Verification items for the finished model (mm, model axes). Face numbers are marked on the shaded views. Round coordinates to 2 decimals unless told otherwise and drop trailing zeros. Loops run counter-clockwise (first coordinate to the right, second up) from the corner with the lowest first, then second, coordinate; pieces in that order, holes last. Notation, with made-up numbers: M -32,24 L 6,24 A19 ccw 6,35 Z; hole C 39,-28 d6. An arc over 180 degrees is marked long. One line per item, written item: value.
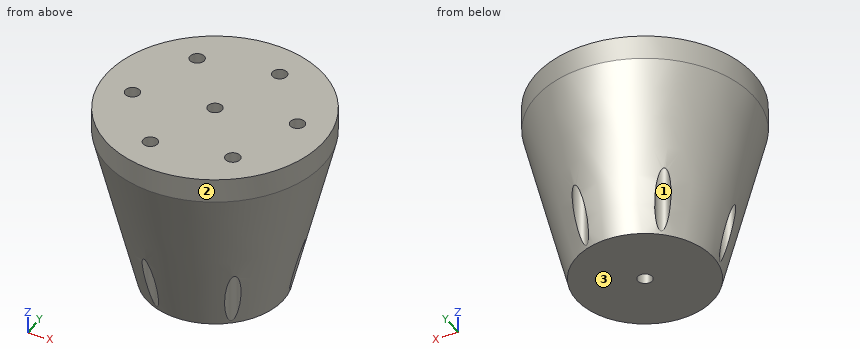
from build123d import *

# Parameters (mm, degrees)
F0_R     = 13.5
F0_R_2   = 0.9
F1_DEPTH = 23


# Not quite as in the source:
# - a fillet or chamfer that OpenCascade refuses, or shapes differently, is made with other operations: its cross-section is extruded or revolved along the edge and cut away or added


with BuildPart() as f1:
    # F0 (on Top) → F1 (new body)
    with BuildSketch(Plane.XY):
        Circle(F0_R)
        with Locations((-3.1211513103, -8.9726481319)):
            Circle(F0_R_2, mode=Mode.SUBTRACT)
        with Locations((-9.3311168766, -1.7833277421)):
            Circle(F0_R_2, mode=Mode.SUBTRACT)
        with Locations((6.2099655662, -7.1893203897)):
            Circle(F0_R_2, mode=Mode.SUBTRACT)
        with Locations((-6.2099655662, 7.1893203897)):
            Circle(F0_R_2, mode=Mode.SUBTRACT)
        Circle(F0_R_2, mode=Mode.SUBTRACT)
        with Locations((9.3311168766, 1.7833277421)):
            Circle(F0_R_2, mode=Mode.SUBTRACT)
        with Locations((3.1211513103, 8.9726481319)):
            Circle(F0_R_2, mode=Mode.SUBTRACT)
    extrude(amount=F1_DEPTH)

    # F2: chamfer of 20 x 5 on 1 edges, made by hand

    # F2_s1 → F2_t2 (revolve, cut)
    with BuildSketch(Plane.XZ):
        Polygon((13.5, 20), (8.5, 0), (13.5, 0), align=None)
    revolve(axis=Axis((0, 0, 0), (0, 0, 1)), mode=Mode.SUBTRACT)


solid = f1.part
(1) Mould release check, pull along Y, two halves, no side actions. Record for the marked faces 1, 2 and 3: +Y half, -Y half, draft (parallel to the pull), parting line (faces both ways), or undercut.
Completed:
face 1: undercut
face 2: parting line
face 3: draft
(2) Depth check by flat-ended pin: pin 1 Ø1.4 at (x, y) = (3.12, 8.97) entering from +Z; pin 2 Ø1.5 at (y, z) = (0.5, 19) entering from +X; pin 3 Ø2.5 at (x, y) = (-6.21, 7.19) entering from +Z; pin 4 Ø4 at (x, z) = (1.5, 4.5) entering from +Y. Enter the tip coordinate at first touch or a pass-through.
Completed:
pin 1: passes through
pin 2: stops at x = 13.43
pin 3: stops at z = 23
pin 4: stops at y = 10.06
(3) Sectioned sample at D-D on z = 14. Enter the section's corners in (x, y), and give its area (3 significant figures).
Completed:
outline: C 0,0 d24; hole C -9.33,-1.78 d1.8; hole C -6.21,7.19 d1.8; hole C -3.12,-8.97 d1.8; hole C 0,0 d1.8; hole C 3.12,8.97 d1.8; hole C 6.21,-7.19 d1.8; hole C 9.33,1.78 d1.8
area: 435 mm^2
(4) Sectioned sample at C-C on z = 5.75. Enter the section's corners in (x, y) (1 decimal), and give its area (3 significant figures).
Completed:
outline: M -9.9,-1.1 A0.9 cw long -9.6,-2.6 A9.9 ccw -4,-9.1 A0.9 cw long -2.5,-9.6 A9.9 ccw 5.9,-8 A0.9 cw long 7.1,-7 A9.9 ccw 9.9,1.1 A0.9 cw long 9.6,2.6 A9.9 ccw 4,9.1 A0.9 cw long 2.5,9.6 A9.9 ccw -5.9,8 A0.9 cw long -7.1,7 A9.9 ccw Z; hole C 0,0 d1.8
area: 296 mm^2
(5) Sectioned sample at A-A on x = 0. Enter the section's corners in (y, z), and give its area (3 significant figures).
Completed:
outline: M -13.5,20 L -8.5,0 L -0.9,0 L -0.9,23 L -13.5,23 Z; M 0.9,0 L 8.5,0 L 13.5,20 L 13.5,23 L 0.9,23 Z
area: 480 mm^2
(6) Thickness scan on L1, parallel to Y at x = 0, z = 18; L2, parallel to X at y = -6.5, z = 16.5; L3, parallel to Y at x = 6.25, z = 17.5. Record the ranges inside material, lowest first. Write a range as from..to.
Completed:
L1: y = -13..-0.9, 0.9..13
L2: x = -10.82..5.63, 6.79..10.82
L3: y = -11.26..-8.09, -6.29..11.26
